```python
from build123d import *

# Parameters (mm, degrees)
SKETCH1_R                       = 1.016
BOSS_EXTRUDE1_DEPTH             = 2
BOSS_EXTRUDE2_OUTLINE_R         = 4.7
BOSS_EXTRUDE2_DEPTH             = 3
BOSS_EXTRUDE5_DEPTH             = 8
BOSS_EXTRUDE6_REACH             = 45.699
BOSS_EXTRUDE6_DIRECTION_2_REACH = 45.699
SKETCH4_W                       = 22.5
SKETCH4_H                       = 14.127681706
CUT_EXTRUDE1_DEPTH              = 7
FILLET1_R                       = 0.5
SKETCH5_R                       = 2.5
BOSS_EXTRUDE7_DEPTH             = 1
SKETCH6_W                       = 5.313656685
SKETCH6_H                       = 4.599259183
SKETCH6_W_2                     = 16.163165117
SKETCH6_H_2                     = 5.344557169
CUT_EXTRUDE2_DEPTH              = 5


# Read off the part's stored shape, not the designer's step: Boss-Extrude2
with BuildPart() as part:
    # Sketch1 → Boss-Extrude1 (new body)
    # profile 1 of 4: a face of its own
    with BuildSketch(Plane.XY):
        with BuildLine():
            Line((-16.05, 5.25), (-16.05, -5.25))
            ThreePointArc((-16.05, -5.25), (-15.801040764, -5.851040764), (-15.2, -6.1))
            Line((-15.2, -6.1), (-11.25, -6.1))
            Line((-11.25, -6.1), (-11.25, 6.1))
            Line((-11.25, 6.1), (-15.2, 6.1))
            ThreePointArc((-15.2, 6.1), (-15.801040764, 5.851040764), (-16.05, 5.25))
        make_face()
        with Locations((-13.9, 0)):
            Circle(SKETCH1_R, mode=Mode.SUBTRACT)
    # profile 2 of 4: a face of its own
    with BuildSketch(Plane.XY):
        with BuildLine():
            Line((16.05, 5.25), (16.05, -5.25))
            ThreePointArc((16.05, -5.25), (15.801040764, -5.851040764), (15.2, -6.1))
            Line((15.2, -6.1), (11.25, -6.1))
            Line((11.25, -6.1), (11.25, 6.094097151))
            Line((11.25, 6.094097151), (15.2, 6.1))
            ThreePointArc((15.2, 6.1), (15.801040764, 5.851040764), (16.05, 5.25))
        make_face()
        with Locations((13.9, 0)):
            Circle(SKETCH1_R, mode=Mode.SUBTRACT)
    # profile 3 of 4: a face of its own
    with BuildSketch(Plane.XY):
        with BuildLine():
            ThreePointArc((15.2, -6.1), (15.801040764, -5.851040764), (16.05, -5.25))
            Line((16.05, -5.25), (16.05, -6.1))
            Line((16.05, -6.1), (15.2, -6.1))
        make_face()
    # profile 4 of 4: a face of its own
    with BuildSketch(Plane.XY):
        with BuildLine():
            ThreePointArc((-16.05, -5.25), (-15.801040764, -5.851040764), (-15.2, -6.1))
            Line((-15.2, -6.1), (-16.05, -6.1))
            Line((-16.05, -6.1), (-16.05, -5.25))
        make_face()
    extrude(amount=BOSS_EXTRUDE1_DEPTH)

    # Boss-Extrude2 outline → Boss-Extrude2 (add)
    with BuildSketch(Plane.XZ.offset(6.1)):
        Polygon((-16.05, 2), (-16.05, 0), (-1.65, 0), (-1.65, -31.072136217), (11.25, -31.072136217), (11.25, 0), (16.05, 0), (16.05, 2), (11.25, 2), (11.25, 24.675592953), (-1.65, 19.952742461), (-1.65, 2), align=None)
        with Locations((4.75, -19)):
            Circle(BOSS_EXTRUDE2_OUTLINE_R, mode=Mode.SUBTRACT)
    extrude(amount=BOSS_EXTRUDE2_DEPTH)

    # Sketch2<3> → Boss-Extrude5 (add)
    with BuildSketch(Plane.XZ.offset(6.1)):
        with BuildLine():
            Line((-1.65, 19.952742461), (-1.65, 16.386819499))
            ThreePointArc((-1.65, 16.386819499), (-0.390222028, 17.279485189), (0.991848608, 17.967797132))
            Line((0.991848608, 17.967797132), (11.246245603, 22.12156627))
            Line((11.246245603, 22.12156627), (11.25, 22.341096015))
            Line((11.25, 22.341096015), (11.25, 24.675592953))
            Line((11.25, 24.675592953), (-1.65, 19.952742461))
        make_face()
        with BuildLine():
            ThreePointArc((4.75, -29.01), (1.347387634, -28.413943333), (-1.65, -26.696759058))
            Line((-1.65, -26.696759058), (-1.65, -31.072136217))
            Line((-1.65, -31.072136217), (11.25, -31.072136217))
            Line((11.25, -31.072136217), (11.25, -28.899497484))
            ThreePointArc((11.25, -28.899497484), (10.201440757, -28.982355275), (9.149976222, -29.01))
            Line((9.149976222, -29.01), (4.75, -29.01))
        make_face()
    extrude(amount=BOSS_EXTRUDE5_DEPTH)

    # Boss-Extrude6: up to this face of the body (flat: up to its plane)
    boss_extrude6_end = Plane(part.part.faces().sort_by_distance((16.05, -1.925, 1))[0])
    # Sketch3 → Boss-Extrude6 (add, up to the picked face)
    with BuildSketch(Plane(origin=(11.25, 0, 0), x_dir=(0, 0, -1), z_dir=(1, 0, 0)), mode=Mode.PRIVATE) as boss_extrude6_sk1:
        Polygon((-7.665828596, -9.1), (-2, -3.457464127), (-2, -9.1), align=None)
    boss_extrude6_tool1 = split(extrude(boss_extrude6_sk1.sketch, amount=BOSS_EXTRUDE6_REACH, mode=Mode.PRIVATE), bisect_by=boss_extrude6_end, keep=Keep.BOTH, mode=Mode.PRIVATE)
    add(boss_extrude6_tool1.solids().sort_by(Axis((11.25, -7.219155, 3.88861), (1, 0, 0)))[0])

    # Boss-Extrude6 direction 2: up to this face of the body (flat: up to its plane)
    boss_extrude6_direction_2_end = Plane(part.part.faces().sort_by_distance((-16.05, -1.925, 1))[0])
    # Sketch3 → Boss-Extrude6 direction 2 (add, up to the picked face)
    with BuildSketch(Plane(origin=(11.25, 0, 0), x_dir=(0, 0, -1), z_dir=(1, 0, 0)), mode=Mode.PRIVATE) as boss_extrude6_direction_2_sk1:
        Polygon((-7.665828596, -9.1), (-2, -3.457464127), (-2, -9.1), align=None)
    boss_extrude6_direction_2_tool1 = split(extrude(boss_extrude6_direction_2_sk1.sketch, amount=-BOSS_EXTRUDE6_DIRECTION_2_REACH, mode=Mode.PRIVATE), bisect_by=boss_extrude6_direction_2_end, keep=Keep.BOTH, mode=Mode.PRIVATE)
    add(boss_extrude6_direction_2_tool1.solids().sort_by(Axis((11.25, -7.219155, 3.88861), (-1, 0, 0)))[0])

    # Sketch4 → Cut-Extrude1 (cut)
    with BuildSketch(Plane(origin=(0, -6.1, 0), x_dir=(1, 0, 0), z_dir=(0, 1, 0))):
        with Locations((0, -7.063840853)):
            Rectangle(SKETCH4_W, SKETCH4_H)
    extrude(amount=CUT_EXTRUDE1_DEPTH, mode=Mode.SUBTRACT)

    # Fillet1
    fillet1_edges = [part.edges().sort_by_distance(p)[0] for p in [
        (13.65, -9.1, 7.665828596),
        (-8.85, -9.1, 7.665828596),
    ]]
    fillet(fillet1_edges, radius=FILLET1_R)

    # Sketch5 → Boss-Extrude7 (add)
    with BuildSketch(Plane.XZ.offset(9.1)):
        with BuildLine():
            Line((-1.65, 16.386819499), (-1.65, 6.455196792))
            Line((-1.65, 6.455196792), (-16.05, 6.455196792))
            Line((-16.05, 6.455196792), (-16.05, 0))
            Line((-16.05, 0), (-1.65, 0))
            Line((-1.65, 0), (-1.65, -26.696759058))
            ThreePointArc((-1.65, -26.696759058), (1.347387634, -28.413943333), (4.75, -29.01))
            Line((4.75, -29.01), (9.149976222, -29.01))
            ThreePointArc((9.149976222, -29.01), (10.201440757, -28.982355275), (11.25, -28.899497484))
            Line((11.25, -28.899497484), (11.25, 0))
            Line((11.25, 0), (16.05, 0))
            Line((16.05, 0), (16.05, 6.455196792))
            Line((16.05, 6.455196792), (11.25, 6.455196792))
            Line((11.25, 6.455196792), (11.25, 22.341096015))
            Line((11.25, 22.341096015), (11.246245603, 22.12156627))
            Line((11.246245603, 22.12156627), (0.991848608, 17.967797132))
            ThreePointArc((0.991848608, 17.967797132), (-0.390222028, 17.279485189), (-1.65, 16.386819499))
        make_face()
        with Locations((4.75, -19)):
            Circle(SKETCH5_R, mode=Mode.SUBTRACT)
    extrude(amount=BOSS_EXTRUDE7_DEPTH)

    # Sketch6 → Cut-Extrude2 (cut)
    with BuildSketch(Plane.XY.offset(6.455196792)):
        with Locations((13.906828343, -7.800370409)):
            Rectangle(SKETCH6_W, SKETCH6_H)
        with Locations((-9.731582558, -7.427721416)):
            Rectangle(SKETCH6_W_2, SKETCH6_H_2)
    extrude(amount=CUT_EXTRUDE2_DEPTH, mode=Mode.SUBTRACT)


solid = part.part
```
CAD build for the part. Positions are in the model's coordinates, mm. A direction names the side the tool comes from. Coordinates: 2 decimals unless noted, no trailing zeros. Order: outer loops, then holes, each group sorted by start corner. A loop starts at its lowest first (then second) coordinate and runs counter-clockwise, first axis right, second up. Notation, with made-up numbers: (14, -6) - (59, -6) arc R6 cw to (59, 0) - close; hole circle Ø4 at (53, -32). An arc over 180 degrees is marked (long way). Answer in a Markdown table with one row per item.
1. Drill centre lines: L1, parallel to X at y = -2.75, z = 1; L2, parallel to Y at x = 7, z = 20; L3, parallel to Z at x = 14.5, y = 3. Where is each one in solid material? Low to high. Write a range as from..to.
Answer:
| item | result |
|---|---|
| L1 | -16.05..-11.25, 11.25..16.05 |
| L2 | -10.1..-6.1 |
| L3 | 0..2 |
2. Slice it at D-D, the plane z = -19. List the corners of the cut face in (x, y), then the cut area to 3 significant figures.
Answer:
| item | result |
|---|---|
| outline | (-1.65, -10.1) - (2.25, -10.1) - (2.25, -9.1) - (0.05, -9.1) - (0.05, -6.1) - (-1.65, -6.1) - close; (7.25, -10.1) - (11.25, -10.1) - (11.25, -6.1) - (9.45, -6.1) - (9.45, -9.1) - (7.25, -9.1) - close |
| area | 18.4 mm² |
3. 3-axis set-ups, long thin cutter, end or side, ignore diameter. For faces 1 (the face through (-13.6, 1.4, 2)), 2 (the face through (14, -9, 6.455)), 3 (the face through (3.73, -7.58, -23.59)), 4 (the face through (11.25, -8, -16)), 5 (the face through (11.25, 0, 1)): which of +Z, -Z, +X, -X, +Y, -Y reach the whole face in a straight line?
Answer:
| item | result |
|---|---|
| face 1 | +Z, +X, -X, +Y |
| face 2 | +Z, +X, +Y, -Y |
| face 3 | +Y |
| face 4 | -Z, +X, +Y, -Y |
| face 5 | +Z, -Z, +Y |
4. Slice it at B-B, the plane x = -13.9. List the corners of the cut face in (y, z), then the cut area to 3 significant figures.
Answer:
| item | result |
|---|---|
| outline | (-10.1, 0) - (-1.02, 0) - (-1.02, 2) - (-3.46, 2) - (-7.89, 6.46) - (-10.1, 6.46) - close; (1.02, 0) - (6.1, 0) - (6.1, 2) - (1.02, 2) - close |
| area | 48.0 mm² |
5. Slice it at C-C, the plane y = 0. List the corners of the cut face in (x, z).
Answer:
| item | result |
|---|---|
| outline | (-16.05, 0) - (-14.92, 0) - (-14.92, 2) - (-16.05, 2) - close; (-12.88, 0) - (-11.25, 0) - (-11.25, 2) - (-12.88, 2) - close; (11.25, 0) - (12.88, 0) - (12.88, 2) - (11.25, 2) - close; (14.92, 0) - (16.05, 0) - (16.05, 2) - (14.92, 2) - close |
6. Pull direction X, two halves, no side cores. Call faces 6 (the face through (13.7, 1.4, 2)), 7 (the face through (6.047, -12.072, 20.016)), 8 (the face through (1.39, -12.07, -28.43)): +X half, -X half, draft (parallel to the pull), parting line (faces both ways), or undercut.
Answer:
| item | result |
|---|---|
| face 6 | draft |
| face 7 | +X half |
| face 8 | undercut |
7. Flat gauge pins, fed straight in: P1, Ø1.1, axis at x = 14.5, y = -9, coming from the +Z side; P2, Ø12, axis at x = 2, y = -9, coming from the +Z side; P3, Ø2.5, axis at x = 14.5, y = 1, coming from the +Z side. Where does each tip first touch, or does it go through?
Answer:
| item | result |
|---|---|
| P1 | z = 6.46 |
| P2 | z = 23.49 |
| P3 | z = 2 |
8. Slice it at A-A, the plane y = -10.75. List the corners of the cut face in (x, z), then the cut area to 3 significant figures.
Answer:
| item | result |
|---|---|
| outline | (-1.65, -31.07) - (11.25, -31.07) - (11.25, -28.9) arc R20.01 cw to (9.15, -29.01) - (4.75, -29.01) arc R10.01 cw to (-1.65, -26.7) - close; (-1.65, 16.39) arc R10.01 cw to (0.99, 17.97) - (11.25, 22.12) - (11.25, 22.34) - (11.25, 24.68) - (-1.65, 19.95) - close |
| area | 68.0 mm² |
